Geometry: final body of the model. Coordinates: model frame, mm. A direction names the side the tool comes from. Round coordinates to 2 decimals unless told otherwise and drop trailing zeros. Write each loop counter-clockwise with the first axis right and the second up, starting at its lowest first coordinate (ties: lowest second). Pieces come first, ordered by that corner, then holes. Notation, with made-up numbers: M -8,37.25 L 0,37.25 A14 ccw 0,56.25 Z; hole C -10,38 d6. An arc over 180 degrees is marked long. Use one line per item in the form item = value. Start each with the question number.
from build123d import *

# Parameters (mm, degrees)
SKETCH1_W           = 25
SKETCH1_H           = 25
SKETCH1_W_2         = 22.500853306
SKETCH1_H_2         = 22.500853306
BOSS_EXTRUDE1_DEPTH = 15
SKETCH2_R           = 1.5
CUT_EXTRUDE1_DEPTH  = 32.721443851
SKETCH3_R           = 1.5
CUT_EXTRUDE2_DEPTH  = 32.721443851


with BuildPart() as part:
    # Sketch1 → Boss-Extrude1 (new body)
    with BuildSketch(Plane(origin=(0, 0, 0), x_dir=(1, 0, 0), z_dir=(0, 1, 0))):
        Rectangle(SKETCH1_W, SKETCH1_H)
        Rectangle(SKETCH1_W_2, SKETCH1_H_2, mode=Mode.SUBTRACT)
    extrude(amount=BOSS_EXTRUDE1_DEPTH)

    # Sketch2 → Cut-Extrude1 (cut, through all)
    with BuildSketch(Plane(origin=(0, 0, -12.5), x_dir=(-1, 0, 0), z_dir=(0, 0, -1))):
        with Locations((0, 7.5)):
            Circle(SKETCH2_R)
    extrude(amount=-CUT_EXTRUDE1_DEPTH, mode=Mode.SUBTRACT)

    # Sketch3 → Cut-Extrude2 (cut, through all)
    with BuildSketch(Plane(origin=(12.5, 0, 0), x_dir=(0, 0, -1), z_dir=(1, 0, 0))):
        with Locations((0, 7.5)):
            Circle(SKETCH3_R)
    extrude(amount=-CUT_EXTRUDE2_DEPTH, mode=Mode.SUBTRACT)


solid = part.part
1. Section query A-A (y = 7.5). Return loops of the section in (x, z), then the cut area to 3 significant figures.
2. Ray query, probe 1 along X at (y, z) = (12, 5); probe 2 along Y at (x, z) = (0, 12). Return the intervals inside material, ascending.
3. Section query D-D (z = 6.5). Return loops of the section in (x, y).
4. Section query C-C (z = 0). Return loops of the section in (x, y), then the cut area to 3 significant figures.
5. Contact query for a flat-ended pin moving along its axis: pin 1 (10 mm diameter, centred on x = 5.5, z = -6, fed in from +Y). Output: stop coordinate, or through.
6. Set-up query: faces 1 (the face through (12.5, 5.7, 0.2)), 2 (the face through (-0.2, 5.7, 11.25)). Return all of +Z, -Z, +X, -X, +Y, -Y with unobstructed straight access to the full face (end or side cutting, diameter ignored); none if empty.
7. Pull-direction query (Y, two-part tool) for faces 3 (the face through (-12, 6, 0)), 4 (the face through (-1, 0, 12)), 5 (the face through (11.25, 5.7, 0.2)); classes: released by +Y, released by -Y, zero draft, split by the parting line, or undercut.
8. Section query B-B (x = -4.25). Return loops of the section in (y, z).
Checks:
q1.outline = M -12.5,-12.5 L -1.5,-12.5 L -1.5,-11.25 L -11.25,-11.25 L -11.25,-1.5 L -12.5,-1.5 Z; M -12.5,1.5 L -11.25,1.5 L -11.25,11.25 L -1.5,11.25 L -1.5,12.5 L -12.5,12.5 Z; M 1.5,-12.5 L 12.5,-12.5 L 12.5,-1.5 L 11.25,-1.5 L 11.25,-11.25 L 1.5,-11.25 Z; M 1.5,11.25 L 11.25,11.25 L 11.25,1.5 L 12.5,1.5 L 12.5,12.5 L 1.5,12.5 Z
q1.area = 104 mm^2
q2.probe_1 = -12.5 to -11.25, 11.25 to 12.5
q2.probe_2 = 0 to 6, 9 to 15
q3.outline = M -12.5,0 L -11.25,0 L -11.25,15 L -12.5,15 Z; M 11.25,0 L 12.5,0 L 12.5,15 L 11.25,15 Z
q4.outline = M -12.5,0 L -11.25,0 L -11.25,6 L -12.5,6 Z; M -12.5,9 L -11.25,9 L -11.25,15 L -12.5,15 Z; M 11.25,0 L 12.5,0 L 12.5,6 L 11.25,6 Z; M 11.25,9 L 12.5,9 L 12.5,15 L 11.25,15 Z
q4.area = 30.0 mm^2
q5.pin_1 = through
q6.face_1 = +Z, -Z, +X, +Y, -Y
q6.face_2 = +Y, -Y
q7.face_3 = undercut
q7.face_4 = released by -Y
q7.face_5 = zero draft
q8.outline = M 0,-12.5 L 15,-12.5 L 15,-11.25 L 0,-11.25 Z; M 0,11.25 L 15,11.25 L 15,12.5 L 0,12.5 Z
